from build123d import *

# Parameters (mm, degrees)
SKETCH1_W           = 30
SKETCH1_H           = 30
BOSS_EXTRUDE1_DEPTH = 2.5
SKETCH2_R           = 5
CUT_EXTRUDE1_DEPTH  = 2.5
SKETCH4_W           = 2
SKETCH4_H           = 30
BOSS_EXTRUDE2_DEPTH = 31.75
SKETCH5_R           = 2.5
CUT_EXTRUDE2_DEPTH  = 30.75
CUT_EXTRUDE3_DEPTH  = 30.75


with BuildPart() as part:
    # Sketch1 → Boss-Extrude1 (new body)
    with BuildSketch(Plane(origin=(0, 0, 0), x_dir=(1, 0, 0), z_dir=(0, 1, 0))):
        Rectangle(SKETCH1_W, SKETCH1_H)
    extrude(amount=BOSS_EXTRUDE1_DEPTH)

    # Sketch2 → Cut-Extrude1 (cut)
    with BuildSketch(Plane(origin=(0, 2.5, 0), x_dir=(1, 0, 0), z_dir=(0, 1, 0))):
        with Locations((0, 5)):
            Circle(SKETCH2_R)
    extrude(amount=-CUT_EXTRUDE1_DEPTH, mode=Mode.SUBTRACT)

    # Sketch4 → Boss-Extrude2 (add)
    with BuildSketch(Plane(origin=(0, 2.5, 0), x_dir=(1, 0, 0), z_dir=(0, 1, 0))):
        with Locations((-14, 0)):
            Rectangle(SKETCH4_W, SKETCH4_H)
        with Locations((14, 0)):
            Rectangle(SKETCH4_W, SKETCH4_H)
    extrude(amount=BOSS_EXTRUDE2_DEPTH)

    # Sketch5 → Cut-Extrude2 (cut)
    with BuildSketch(Plane.ZY.offset(15)):
        with Locations((0, 21.75)):
            Circle(SKETCH5_R)
    extrude(amount=-CUT_EXTRUDE2_DEPTH, mode=Mode.SUBTRACT)

    # Sketch6 → Cut-Extrude3 (cut)
    with BuildSketch(Plane.ZY.offset(15)):
        with BuildLine():
            Line((-15, 0), (-7.505901536, 24.085434897))
            ThreePointArc((-7.505901536, 24.085434897), (0, 29.610840542), (7.505901536, 24.085434897))
            Line((7.505901536, 24.085434897), (15, 0))
            Line((15, 0), (15, 34.25))
            Line((15, 34.25), (-15, 34.25))
            Line((-15, 34.25), (-15, 0))
        make_face()
    extrude(amount=-CUT_EXTRUDE3_DEPTH, mode=Mode.SUBTRACT)


solid = part.part
The model under review builds one solid part; all positions refer to its coordinate system, in mm. A direction names the side the tool comes from. Give positions to 0.01 mm unless a question says otherwise; leave off trailing zeros. Write each loop counter-clockwise with the first axis right and the second up, starting at its lowest first coordinate (ties: lowest second). Pieces come first, ordered by that corner, then holes. Notation, with made-up numbers: M 9.5,22 L 42.5,22 A31 cw 42.5,56 Z; hole C 27,25.5 d5. An arc over 180 degrees is marked long. One line per question, with ' | ' between items. Start each with the question number.
Item 1: For faces 1 (the flat face through (-1.181, 2.286, 14.289)), 2 (the flat face through (0, 2.5, 3)), list the 3-axis set-ups (+Z, -Z, +X, -X, +Y, -Y) from which the entire face can be reached by the end or side of a thin tool; tool diameter is ignored.
Item 2: We need section B-B on z = -5. Write out the cut boundary in (x, y), plus the area to 3 significant figures.
Item 3: We need section D-D on z = -2. Write out the cut boundary in (x, y), plus the area to 3 significant figures.
Item 4: Wall thickness on line 1 (X direction, y = 10.5, z = 4.25); line 2 (Y direction, x = -13.35, z = 0); line 3 (X direction, y = 1.45, z = -5): over which ranges is each line inside the solid? List them lowest first. Write a range as from..to.
Item 5: Draft analysis for pull direction Z (two halves, no side actions). For faces 3 (the cylindrical face through (-14.01, 24.23, -0.33)), 4 (the cylindrical face through (-14.01, 29.61, -0.14)), 5 (the flat face through (15, 11, 0)), state which applies: released by +Z, released by -Z, zero draft, split by the parting line, or undercut.
Item 6: We need section C-C on y = 7.5. Write out the cut boundary in (x, z), plus the area to 3 significant figures.
Item 7: For pin 1 (1.5 mm diameter, centred on x = -6, z = -6, fed in from +Y); pin 2 (4 mm diameter, centred on y = 21.75, z = 0, fed in from -X), all flat-tipped, find the tip position at first contact; note any pin that passes through.
Item 8: We need section A-A on x = 3. Write out the cut boundary in (y, z), plus the area to 3 significant figures.
Results found:
1) face 1: +Z, +X, -X, +Y | face 2: +Z, -Z, +Y
2) outline: M -15,0 L -5,0 L -5,2.5 L -13,2.5 L -13,27.82 L -15,27.82 Z; M 5,0 L 15,0 L 15,27.82 L 13,27.82 L 13,2.5 L 5,2.5 Z | area: 151 mm2
3) outline: M -15,0 L -4,0 L -4,2.5 L -13,2.5 L -13,20.25 L -15,20.25 Z; M -15,23.25 L -13,23.25 L -13,29.35 L -15,29.35 Z; M 4,0 L 15,0 L 15,20.25 L 13,20.25 L 13,2.5 L 4,2.5 Z; M 13,23.25 L 15,23.25 L 15,29.35 L 13,29.35 Z | area: 150 mm2
4) line 1: x = -15..-13, 13..15 | line 2: y = 0..19.25, 24.25..29.61 | line 3: x = -15..-5, 5..15
5) face 3: undercut | face 4: split by the parting line | face 5: zero draft
6) outline: M -15,-12.67 L -13,-12.67 L -13,12.67 L -15,12.67 Z; M 13,-12.67 L 15,-12.67 L 15,12.67 L 13,12.67 Z | area: 101 mm2
7) pin 1: stops at y = 2.5 | pin 2: passes through
8) outline: M 0,-15 L 2.5,-14.22 L 2.5,-9 L 0,-9 Z; M 0,-1 L 2.5,-1 L 2.5,14.22 L 0,15 Z | area: 53.1 mm2
